Part model, mm, in its own coordinate system. Face numbers are marked on the shaded views. A direction names the side the tool comes from. Round coordinates to 2 decimals unless told otherwise and drop trailing zeros. Write each loop counter-clockwise with the first axis right and the second up, starting at its lowest first coordinate (ties: lowest second). Pieces come first, ordered by that corner, then holes.
```python
from build123d import *

# Parameters (mm, degrees)
SKETCH_1_W          = 120
SKETCH_1_H          = 120
EXTRUDE_1_DEPTH     = 86.5
SKETCH_2_R          = 55
EXTRUDE_2_DEPTH     = 5
SKETCH_3_R          = 38.5
EXTRUDE_3_DEPTH     = 5.5
SKETCH_4_R          = 9.5
EXTRUDE_4_DEPTH     = 29.5
SKETCH_5_R          = 5
CUT_EXTRUDE_1_DEPTH = 191.479001467
CUT_EXTRUDE_2_DEPTH = 76.5
FILLET_1_R          = 3


with BuildPart() as part:
    # 草图1 → 拉伸1 (new body)
    with BuildSketch(Plane.XY):
        with Locations((60, -60)):
            Rectangle(SKETCH_1_W, SKETCH_1_H)
    extrude(amount=EXTRUDE_1_DEPTH)

    # 草图2 → 拉伸2 (add)
    with BuildSketch(Plane(origin=(0, 0, 0), x_dir=(-1, 0, 0), z_dir=(0, 0, -1))):
        with Locations(Location((-60, -60, 0), (0, 0, 180))):
            Circle(SKETCH_2_R)
    extrude(amount=EXTRUDE_2_DEPTH)

    # 草图3 → 拉伸3 (add)
    with BuildSketch(Plane(origin=(0, 0, -5), x_dir=(-1, 0, 0), z_dir=(0, 0, -1))):
        with Locations((-60, -60)):
            Circle(SKETCH_3_R)
    extrude(amount=EXTRUDE_3_DEPTH)

    # 草图4 → 拉伸4 (add)
    with BuildSketch(Plane(origin=(0, 0, -10.5), x_dir=(-1, 0, 0), z_dir=(0, 0, -1))):
        with Locations((-60, -60)):
            Circle(SKETCH_4_R)
    extrude(amount=EXTRUDE_4_DEPTH)

    # 草图5 → 切除-拉伸1 (cut, through all)
    with BuildSketch(Plane(origin=(0, 0, 0), x_dir=(-1, 0, 0), z_dir=(0, 0, -1))):
        with Locations((-8.734758364, -111.265241636)):
            Circle(SKETCH_5_R)
        with Locations((-8.734758364, -8.734758364)):
            Circle(SKETCH_5_R)
        with Locations((-111.265241636, -111.265241636)):
            Circle(SKETCH_5_R)
        with Locations((-111.265241636, -8.734758364)):
            Circle(SKETCH_5_R)
    extrude(amount=-CUT_EXTRUDE_1_DEPTH, mode=Mode.SUBTRACT)

    # 草图6 → 切除-拉伸2 (cut)
    with BuildSketch(Plane.XY.offset(86.5)):
        with BuildLine():
            Line((8.734758364, -16.734758364), (0, -16.734758364))
            Line((0, -16.734758364), (0, 0))
            Line((0, 0), (16.734758364, 0))
            Line((16.734758364, 0), (16.734758364, -8.734758364))
            ThreePointArc((16.734758364, -8.734758364), (14.391612613, -14.391612613), (8.734758364, -16.734758364))
        make_face()
        with BuildLine():
            Line((111.265241636, -103.265241636), (120, -103.265241636))
            Line((120, -103.265241636), (120, -120))
            Line((120, -120), (103.265241636, -120))
            Line((103.265241636, -120), (103.265241636, -111.265241636))
            ThreePointArc((103.265241636, -111.265241636), (105.608387387, -105.608387387), (111.265241636, -103.265241636))
        make_face()
        with BuildLine():
            Line((120, 0), (103.265241636, 0))
            Line((103.265241636, 0), (103.265241636, -8.734758364))
            ThreePointArc((103.265241636, -8.734758364), (105.608387387, -14.391612613), (111.265241636, -16.734758364))
            Line((111.265241636, -16.734758364), (120, -16.734758364))
            Line((120, -16.734758364), (120, 0))
        make_face()
        with BuildLine():
            Line((0, -120), (16.734758364, -120))
            Line((16.734758364, -120), (16.734758364, -111.265241636))
            ThreePointArc((16.734758364, -111.265241636), (14.391612613, -105.608387387), (8.734758364, -103.265241636))
            Line((8.734758364, -103.265241636), (0, -103.265241636))
            Line((0, -103.265241636), (0, -120))
        make_face()
    extrude(amount=-CUT_EXTRUDE_2_DEPTH, mode=Mode.SUBTRACT)

    # 圆角1
    fillet_1_edges = [part.edges().sort_by_distance(p)[0] for p in [
        (103.265241636, 0, 48.25),
        (120, -16.734758364, 48.25),
        (16.734758364, 0, 48.25),
        (0, -16.734758364, 48.25),
        (120, -103.265241636, 48.25),
        (103.265241636, -120, 48.25),
        (16.734758364, -120, 48.25),
        (0, -103.265241636, 48.25),
    ]]
    fillet(fillet_1_edges, radius=FILLET_1_R)


solid = part.part
```
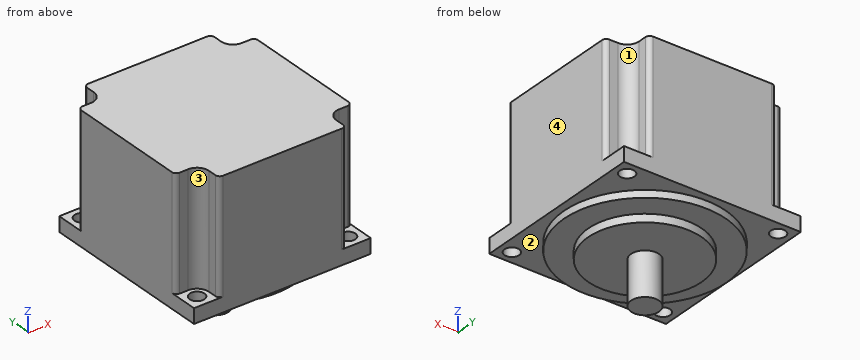
Q1. Which spindle directions (+Z, -Z, +X, -X, +Y, -Y) get a long thin tool onto all of the face, cutting with end or side? Do the marked faces 1, 2, 3 and 4. Say none if no direction does.
Values follow:
face 1: +Z, +X, +Y
face 2: -Z
face 3: +Z, -X, -Y
face 4: +Z, -Z, +X, +Y, -Y
Q2. Drop flat-ended pins along their axis: pin 1 (21.5 mm diameter, centred on x = 113.5, y = -6.5, fed in from +Z); pin 2 (1 mm diameter, centred on x = 76.5, y = -52.5, fed in from -Z); pin 3 (8 mm diameter, centred on x = 15.5, y = -74.5, fed in from -Z); pin 4 (3 mm diameter, centred on y = -105.5, z = 47, fed in from -X). Give the stop position or say it passes through.
Values follow:
pin 1: stops at z = 86.5
pin 2: stops at z = -10.5
pin 3: stops at z = -5
pin 4: stops at x = 12.08
Q3. Cut at C-C on x = 60. Write the cut outline in (y, z), plus the area to 3 significant figures.
Values follow:
outline: (-120, 0) - (-115, 0) - (-115, -5) - (-98.5, -5) - (-98.5, -10.5) - (-69.5, -10.5) - (-69.5, -40) - (-50.5, -40) - (-50.5, -10.5) - (-21.5, -10.5) - (-21.5, -5) - (-5, -5) - (-5, 0) - (0, 0) - (0, 86.5) - (-120, 86.5) - close
area: 11,900 mm2
Q4. Cut at B-B on y = -60. Write the cut outline in (x, z), plus the area to 3 significant figures.
Values follow:
outline: (0, 0) - (5, 0) - (5, -5) - (21.5, -5) - (21.5, -10.5) - (50.5, -10.5) - (50.5, -40) - (69.5, -40) - (69.5, -10.5) - (98.5, -10.5) - (98.5, -5) - (115, -5) - (115, 0) - (120, 0) - (120, 86.5) - (0, 86.5) - close
area: 11,900 mm2
Q5. Cut at D-D on y = -38.5. Write the cut outline in (x, z).
Values follow:
outline: (0, 0) - (9.38, 0) - (9.38, -5) - (28.06, -5) - (28.06, -10.5) - (91.94, -10.5) - (91.94, -5) - (110.62, -5) - (110.62, 0) - (120, 0) - (120, 86.5) - (0, 86.5) - close
Q6. Wall check: L1, parallel to X at y = -108, z = 4; L2, parallel to Z at x = 61, y = -6.5; L3, parallel to X at y = -15, z = 46.5. Give the ranges that are in metal, low to high.
Values follow:
L1: x = 0 to 4.95, 12.52 to 107.48, 115.05 to 120
L2: z = -5 to 86.5
L3: x = 13.71 to 106.29
Q7. Cut at A-A on z = 74. Write the cut outline in (x, y).
Values follow:
outline: (0, -100.27) arc R3 ccw to (3, -103.27) - (8.73, -103.27) arc R8 cw to (16.73, -111.27) - (16.73, -117) arc R3 ccw to (19.73, -120) - (100.27, -120) arc R3 ccw to (103.27, -117) - (103.27, -111.27) arc R8 cw to (111.27, -103.27) - (117, -103.27) arc R3 ccw to (120, -100.27) - (120, -19.73) arc R3 ccw to (117, -16.73) - (111.27, -16.73) arc R8 cw to (103.27, -8.73) - (103.27, -3) arc R3 ccw to (100.27, 0) - (19.73, 0) arc R3 ccw to (16.73, -3) - (16.73, -8.73) arc R8 cw to (8.73, -16.73) - (3, -16.73) arc R3 ccw to (0, -19.73) - close
